Read the model definition and answer for the solid it produces. Units are mm, in the model's axes. A direction names the side the tool comes from. Give positions to 0.01 mm unless a question says otherwise; leave off trailing zeros. Loops run counter-clockwise (first coordinate to the right, second up) from the corner with the lowest first, then second, coordinate; pieces in that order, holes last. Notation, with made-up numbers: (-4.5, 59.5) -> (2.5, 59.5) arc R30 ccw to (2.5, 97.5) -> close; hole circle Ø4 at (-11, -17). An arc over 180 degrees is marked (long way). Answer as CSV lines item,"result". Start each with the question number.
Autodesk Fusion 360 part; units mm, degrees
sketch "Sketch1" plane through (0, 0, 0) normal (0, 1, 0) x (1, 0, 0)
  line L0 (0, 0) -> (7, 0)
  line L1 (7, 0) -> (7, -19)
  line L2 (7, -19) -> (0, -19)
  line L3 (0, -19) -> (0, 0)
  dimension "d1" = 7
  dimension "d2" = 19
extrude "Extrude1" add sketch "Sketch1" along normal blind 4.95
sketch "Sketch3" plane through (0, 4.95, 0) normal (0, 1, 0) x (-1, 0, 0)
  line L0 (0, 19) -> (-7, 19)
  line L1 (-7, 19) -> (-7, 0)
  line L2 (-7, 0) -> (0, 0)
  line L3 (0, 0) -> (0, 19)
  line L4 (0, 0) -> (-2, 0)
  line L5 (-2, 0) -> (-2, 19)
  line L6 (-2, 19) -> (0, 19)
  line L7 (0, 19) -> (0, 0)
  dimension "d8" = 2
extrude "Extrude3" add sketch "Sketch3" along normal blind 6.95 contours L0 L2 L3 L4 L5 L6 L7
ref_plane "WorkPlane1" through (3.5, 5.95, 9.5) normal (0, 0, 1) x (1, 0, 0)
sketch "Sketch4" plane through (0, 0, 19) normal (0, 0, 1) x (1, 0, 0)
  line L0 (0, 0) -> (7, 0)
  line L1 (7, 0) -> (7, 4.95)
  line L2 (7, 4.95) -> (2, 4.95)
  line L3 (2, 4.95) -> (2, 11.9)
  line L4 (2, 11.9) -> (0, 11.9)
  line L5 (0, 11.9) -> (0, 0)
  line L6 (2, 4.95) -> (7, 4.95)
  line L7 (7, 4.95) -> (7, 3.05)
  line L8 (7, 3.05) -> (2, 3.05)
  line L9 (2, 3.05) -> (2, 4.95)
  dimension "d21" = 3.05
extrude "Extrude4" add sketch "Sketch4" along normal blind 8 contours L1 L2 L6 L7 L8 L9
mirror "Mirror1" about plane through (3.5, 5.95, 9.5) normal (0, 0, 1) of "Extrude4"
sketch "Sketch5" plane through (0, 4.95, 0) normal (0, 1, 0) x (-1, 0, 0)
  line L0 (-7, 27) -> (-7, -8)
  line L1 (-7, -8) -> (-2, -8)
  line L2 (-2, -8) -> (-2, 0)
  line L3 (-2, 0) -> (-2, 19)
  line L4 (-2, 19) -> (-2, 27)
  line L5 (-2, 27) -> (-7, 27)
  line L6 (0, 19) -> (-2, 19)
  line L7 (0.7, 9.5) -> (-7.7, 9.5)
  point P0 (-4.5, 23)
  point P1 (-4.5, -4)
  dimension "d14" = 2.5
  dimension "d15" = 2.5
  dimension "d16" = 4
  dimension "d17" = 5
hole "Hole1" at (4.5, 4.95, -4) at (4.5, 4.95, 23) direction (0, -1, 0) diameter 2.4 depth 2 tip angle 118
sketch "Sketch6" plane through (0, 0, 0) normal (0, -1, 0) x (1, 0, 0)
  line L0 (0, 0) -> (7, 0)
  line L1 (7, 0) -> (7, 19)
  line L2 (7, 19) -> (0, 19)
  line L3 (0, 19) -> (0, 0)
  line L4 (3.5, 17.5) -> (5.5, 17.5)
  line L5 (5.5, 17.5) -> (5.5, 1.5)
  line L6 (5.5, 1.5) -> (3.5, 1.5)
  line L7 (3.5, 1.5) -> (3.5, 17.5)
  dimension "d22" = 2
  dimension "d23" = 1.5
  dimension "d24" = 1.5
  dimension "d25" = 1.5
extrude "Extrude5" add sketch "Sketch6" along normal blind 3.5 contours L4 L5 L6 L7
sketch "Sketch7" plane through (5.5, 0, 0) normal (1, 0, 0) x (0, 0, -1)
  line L0 (-1.5, 0) -> (-17.5, 0)
  line L1 (-17.5, 0) -> (-17.5, -3.5)
  line L2 (-17.5, -3.5) -> (-1.5, -3.5)
  line L3 (-1.5, -3.5) -> (-1.5, 0)
  line L4 (-17.5, -3.5) -> (-1.5, -3.5)
  line L5 (-1.5, -3.5) -> (-1.5, -1.5)
  line L6 (-1.5, -1.5) -> (-17.5, -1.5)
  line L7 (-17.5, -1.5) -> (-17.5, -3.5)
  dimension "d28" = 2
sketch "Sketch8" plane through (0, 0, 0) normal (0, 0, 1) x (1, 0, 0)
  line L0 (5.5, -3.6158) -> (45.5, -2.9158)
  line L1 (5.5, -3.5) -> (5.5, -1.5)
  dimension "d29" = 0.7
  dimension "d30" = 40
sweep "Sweep1" add profiles "Sketch7" path "Sketch8" along L0 section 1 contours L1 L2 L3 L4 L5 L6 L7
fillet "Fillet1" radius 1 3 edges at (3.5, 0, 9.5) (4.5, 0, 1.5) (4.5, 0, 17.5)
fillet "Fillet1" radius 1 1 edges at (5.5, 0, 9.5)
fillet "Fillet2" radius 0.6 9 edges at (3.5, -3.5, 9.5) (25.5, -3.15, 1.5) (4.5, -3.5, 1.5) (4.5, -3.5, 17.5) (25.5, -3.15, 17.5) (45.5, -2.8, 9.5) (25.5, -1.15, 1.5) (25.5, -1.15, 17.5) (45.5, -0.8, 9.5)
(1) Each of these flat-tipped pins is pushed along its axis until it touches: P1, Ø5.5, axis at x = 5, z = 24.5, coming from the -Y side; P2, Ø1.9, axis at x = 4.5, z = -4, coming from the -Y side; P3, Ø5.5, axis at x = 2.5, y = 8.5, coming from the -Z side; P4, Ø6, axis at x = 36, z = 19, coming from the -Y side. Where does it stop, or does it pass through?
(2) Find the intervals of material crossed by line 1 along Z through (x, y) = (4.5, 3.6); line 2 along X through (y, z) = (3.8, -4); line 3 along X through (y, z) = (2.75, 6), in increasing order. Write a range as from..to.
(3) Find section A-A on z = -4. Write down the section's boundary in (x, y).
(4) Find section B-B on z = 6. Write down the section's boundary in (x, y), then the cut area to 3 significant figures.
(5) A tool of negligible diameter and unlimited length cuts with its end or side. For faces 4 (the face through (2, 4, 23)), 5 (the face through (6, 3.05, 24)), 6 (the face through (7, 3, 10)), 7 (the face through (25.782, -2.974, 1.68)), from which of +Z, -Z, +X, -X, +Y, -Y can it reach the whole face along a straight path? Write none if from no direction.
(6) Find section D-D on y = 1.25. Write down the section's boundary in (x, z).
(7) Find section C-C on y = 10. Write down the section's boundary in (x, z), then the cut area to 3 significant figures.
(8) The mould has two halves that part along X. Classify faces 1 (the face through (1, 11.9, 10)), 2 (the face through (2, 4, -4)), 3 (the face through (4.45, 3.99, 21.8)): pulls with the +X half, pulls with the -X half, needs draft (parallel to the pull), parting line crosses it, or undercut.
Answer block:
1,P1,"stops at y = 3.05"
1,P2,"passes through"
1,P3,"stops at z = 0"
1,P4,"stops at y = -3"
2,line 1,"z = -8..-5.2, -2.8..21.8, 24.2..27"
2,line 2,"x = 2..3.3, 5.7..7"
2,line 3,"x = 0..7"
3,outline,"(2, 3.05) -> (3.3, 3.05) -> (3.3, 4.95) -> (2, 4.95) -> close; (5.7, 3.05) -> (7, 3.05) -> (7, 4.95) -> (5.7, 4.95) -> close"
4,outline,"(0, 0) -> (2.5, 0) arc R1 cw to (3.5, -1) -> (3.5, -2.9) arc R0.6 ccw to (4.1, -3.5) -> (5.5, -3.5) -> (44.91, -2.81) arc R0.6 ccw to (45.5, -2.21) -> (45.5, -1.41) arc R0.6 ccw to (44.89, -0.81) -> (5.5, -1.5) -> (5.5, -1) arc R1 cw to (6.5, 0) -> (7, 0) -> (7, 4.95) -> (2, 4.95) -> (2, 11.9) -> (0, 11.9) -> close"
4,area,"136 mm2"
5,face 4,"+Z, -X, +Y, -Y"
5,face 5,"+Z, +X, -X, -Y"
5,face 6,"+Z, -Z, +X, +Y"
5,face 7,"-Z, +X, -Y"
6,outline,"(0, 0) -> (7, 0) -> (7, 19) -> (0, 19) -> close"
7,outline,"(0, 0) -> (2, 0) -> (2, 19) -> (0, 19) -> close"
7,area,"38.0 mm2"
8,face 1,"needs draft"
8,face 2,"pulls with the -X half"
8,face 3,"undercut"
